The model under review builds one solid part; all positions refer to its coordinate system, in mm. A direction names the side the tool comes from. Coordinates: 2 decimals unless noted, no trailing zeros. Put each result on its own line as item: value. Start each with the question number.
Item 1: For pin 1 (3 mm diameter, centred on x = -114, y = 97, fed in from +Z); pin 2 (1.6 mm diameter, centred on x = -6, y = -97, fed in from -Z); pin 3 (2.5 mm diameter, centred on x = -114, y = -97, fed in from -Z), all flat-tipped, find the tip position at first contact; note any pin that passes through.
Item 2: Mouldability with a two-part tool opening along Y and no side actions: class faces 1 (the face through (-61, 105, 3)), 2 (the face through (-115, -98, 3)), 3 (the face through (0, -1, 3)) as pulls with the +Y half, pulls with the -Y half, needs draft (parallel to the pull), parting line crosses it, or undercut.
Item 3: Machinability: for faces 4 (the face through (-61, -105, 3)), 5 (the face through (-115, 96, 3)), which of the approach directions +Z, -Z, +X, -X, +Y, -Y give a long, thin tool a straight path to every point of the face, cutting with its end or side? Answer none if there is none.
Item 4: To check wall thickness, follow L1, parallel to Y at x = -114, z = 4.25; L2, parallel to X at y = -97, z = 3.6; L3, parallel to Y at x = -6, z = 2. State the ranges of each line that lie inside material, in increasing order. Write a range as [from, to].
```python
from build123d import *

# Parameters (mm, degrees)
SKETCH1_W           = 120
SKETCH1_H           = 210
BOSS_EXTRUDE1_DEPTH = 6
SKETCH2_R           = 2
CUT_EXTRUDE1_DEPTH  = 3
SKETCH3_R           = 1
CUT_EXTRUDE2_DEPTH  = 3
FILLET1_R           = 0.5


with BuildPart() as part:
    # Sketch1 → Boss-Extrude1 (new body)
    with BuildSketch(Plane.XY):
        with Locations((-60, 0)):
            Rectangle(SKETCH1_W, SKETCH1_H)
    extrude(amount=BOSS_EXTRUDE1_DEPTH)

    # Sketch2 → Cut-Extrude1 (cut)
    with BuildSketch(Plane(origin=(0, 0, 0), x_dir=(-1, 0, 0), z_dir=(0, 0, -1))):
        with Locations((6, 97)):
            Circle(SKETCH2_R)
        with Locations((114, 97)):
            Circle(SKETCH2_R)
        with Locations((6, -97)):
            Circle(SKETCH2_R)
        with Locations((114, -97)):
            Circle(SKETCH2_R)
    extrude(amount=-CUT_EXTRUDE1_DEPTH, mode=Mode.SUBTRACT)

    # Sketch3 → Cut-Extrude2 (cut)
    with BuildSketch(Plane.XY.offset(6)):
        with Locations((-114, 97)):
            Circle(SKETCH3_R)
        with Locations((-6, 97)):
            Circle(SKETCH3_R)
        with Locations((-6, -97)):
            Circle(SKETCH3_R)
        with Locations((-114, -97)):
            Circle(SKETCH3_R)
    extrude(amount=-CUT_EXTRUDE2_DEPTH, mode=Mode.SUBTRACT)

    # Fillet1
    fillet1_edges = [part.edges().sort_by_distance(p)[0] for p in [
        (0, 0, 6),
        (-60, 105, 6),
        (-120, 0, 6),
        (-60, 105, 0),
        (0, 0, 0),
        (-60, -105, 0),
        (-120, 0, 0),
        (-120, 105, 3),
        (0, 105, 3),
        (0, -105, 3),
        (-120, -105, 3),
        (-60, -105, 6),
    ]]
    fillet(fillet1_edges, radius=FILLET1_R)


solid = part.part
```
Report:
1. pin 1: z = 6
1. pin 2: through
1. pin 3: z = 3
2. face 1: pulls with the +Y half
2. face 2: undercut
2. face 3: needs draft
3. face 4: +Z, -Z, +X, -X, -Y
3. face 5: -Z
4. L1: [-105, -98], [-96, 96], [98, 105]
4. L2: [-120, -115], [-113, -7], [-5, 0]
4. L3: [-105, -99], [-95, 95], [99, 105]
